Check sheet for the drawn part. Datum: minimum x, y, z corner. Units: mm. A direction names the side the tool comes from. Round coordinates to 2 decimals unless told otherwise and drop trailing zeros. Write each loop counter-clockwise with the first axis right and the second up, starting at its lowest first coordinate (ties: lowest second). Pieces come first, ordered by that corner, then holes. Notation, with made-up numbers: (86.25, 20) -> (126.25, 20) arc R28 ccw to (126.25, 39) -> close; hole circle Ø10 at (-16.5, 84.5). An arc over 180 degrees is marked (long way). Use a Markdown table: item, result.
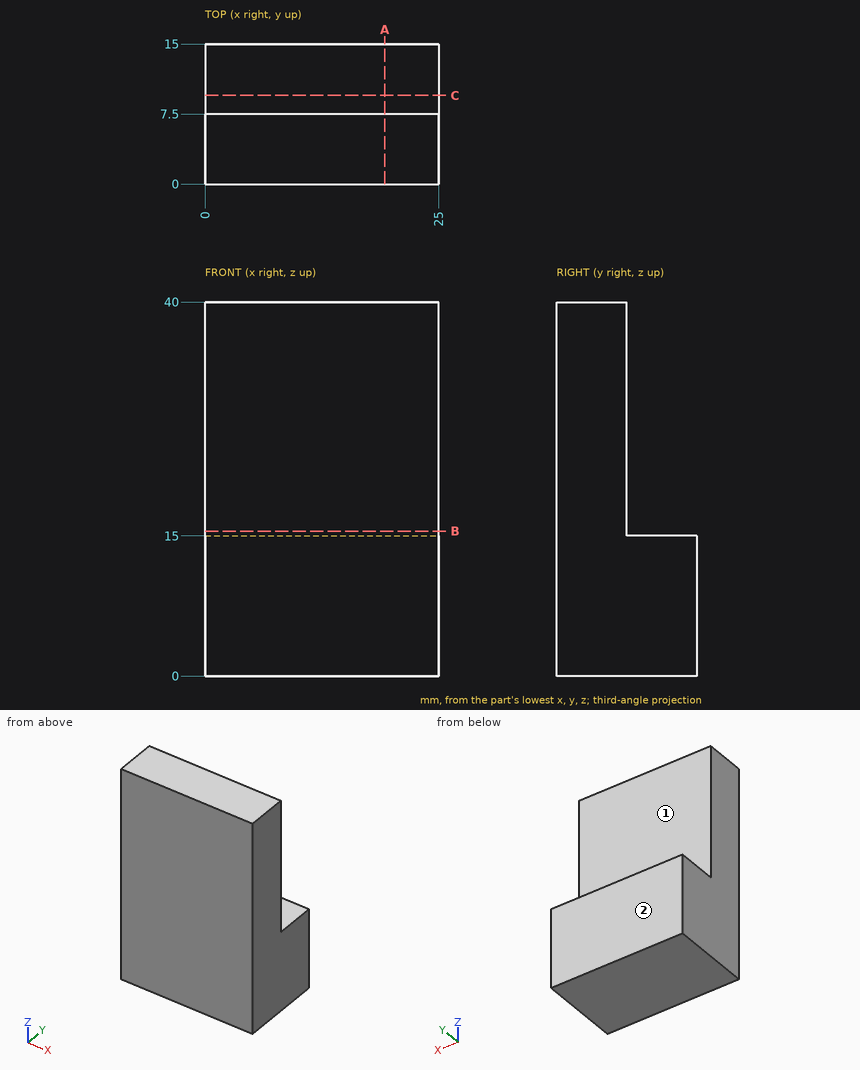
(1) Access from +Z, -Z, +X, -X, +Y, -Y to the whole of each face (thin tool, end or side, straight path). Record for the marked faces 1 and 2.
A:
| item | result |
|---|---|
| face 1 | +Z, +X, -X, +Y |
| face 2 | +Z, -Z, +X, -X, +Y |
(2) Section check B-B on z = 15.5. Record the cut outline in (x, y), plus the area to 4 significant figures.
A:
| item | result |
|---|---|
| outline | (0, 0) -> (25, 0) -> (25, 7.5) -> (0, 7.5) -> close |
| area | 187.5 mm2 |
(3) Thickness scan on line 1 (Z direction, x = 13.75, y = 13.5); line 2 (Y direction, x = 10.25, z = 25). Record the ranges inside material, lowest first.
A:
| item | result |
|---|---|
| line 1 | z = 0 to 15 |
| line 2 | y = 0 to 7.5 |
(4) Section check C-C on y = 9.5. Record the cut outline in (x, z), plus the area to 3 significant figures.
A:
| item | result |
|---|---|
| outline | (0, 0) -> (25, 0) -> (25, 15) -> (0, 15) -> close |
| area | 375 mm2 |
(5) Gauge pin test, flat ends, axial feed: pin 1 Ø4 at (x, y) = (18.5, 13) entering from +Z; pin 2 Ø12.5 at (x, z) = (18.5, 33.5) entering from +Y. Record the tip position at first contact, or that the pin passes through.
A:
| item | result |
|---|---|
| pin 1 | stops at z = 15 |
| pin 2 | stops at y = 7.5 |
(6) Section check A-A on x = 19.25. Record the cut outline in (y, z), plus the area to 4 significant figures.
A:
| item | result |
|---|---|
| outline | (0, 0) -> (15, 0) -> (15, 15) -> (7.5, 15) -> (7.5, 40) -> (0, 40) -> close |
| area | 412.5 mm2 |
